Autodesk Inventor part; units mm, degrees
ref_plane "YZ Plane" through (0, 0, 0) normal (1, 0, 0) x (0, 1, 0)
ref_plane "XZ Plane" through (0, 0, 0) normal (0, 1, 0) x (-1, 0, 0)
ref_plane "XY Plane" through (0, 0, 0) normal (0, 0, 1) x (1, 0, 0)
sketch "Эскиз1" plane through (0, 0, 0) normal (0, 1, 0) x (-1, 0, 0)
  line L0 (7, 44) -> (0, 44)
  line L1 (0, 44) -> (0, 0)
  line L2 (0, 0) -> (7, 0)
  line L3 (7, 0) -> (7, 44)
  line L4 (-16.3445, 0) -> (14.925, 0) construction
  line L5 (0, 24.3748) -> (0, -24.0504) construction
  circle A0 centre (3.5, 39) radius 1.75
  line L6 (3.5, 44) -> (3.5, 0) construction
  line L7 (7, 22) -> (0, 22) construction
  circle A1 centre (3.5, 5) radius 1.75
  point P0 (0, 0)
  dimension "d0" = 44
  dimension "d1" = 7
  dimension "d2" = 3.5
  dimension "d5" = 34
extrude "Выдавливание1" add sketch "Эскиз1" along normal blind 30
sketch "Эскиз2" plane through (0, 0, 44) normal (1, 0, 0) x (0, 0, -1)
  line L0 (0, 0) -> (44, 0) construction
  line L1 (44, 0) -> (44, 30) construction
  line L2 (0, 30) -> (44, 30) construction
  line L3 (0, 0) -> (0, 30) construction
  line L4 (44, 30) -> (0, 30) construction
  line L5 (22, 30) -> (22, 0) construction
  line L6 (44, 0) -> (0, 0) construction
  line L7 (0, 0) -> (0, 30) construction
  line L8 (0, 15) -> (44, 15) construction
  line L9 (44, 0) -> (44, 30) construction
  circle A0 centre (22, 11.2) radius 10.25
  circle A1 centre (22, 11.2) radius 3.75
  circle A2 centre (22, 18.7) radius 1.5
  line L10 (18.25, 11.2) -> (25.75, 11.2) construction
  circle A3 centre (22, 3.7) radius 1.5
  dimension "d8" = 20.5
  dimension "d9" = 11.2
  dimension "d10" = 7.5
  dimension "d11" = 3
  dimension "d12" = 15
extrude "Выдавливание2" cut sketch "Эскиз2" against normal blind 30 contours A1 | A2 | A3
extrude "Выдавливание3" cut sketch "Эскиз2" against normal blind 4
properties part number "motor_front"
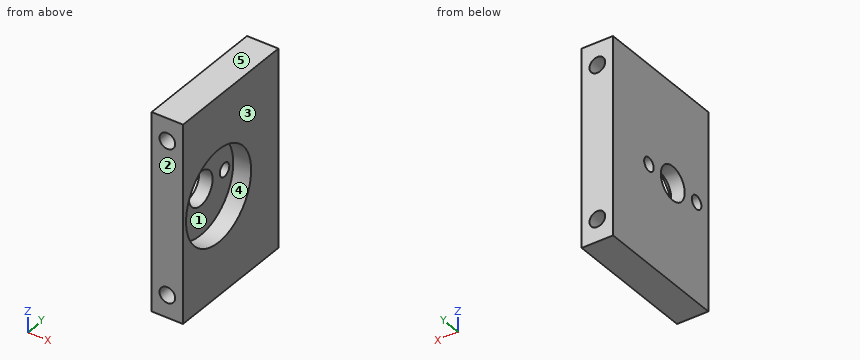
Geometry: final body of the model. Coordinates: model frame, mm. Face numbers are marked on the shaded views. A direction names the side the tool comes from. Give positions to 0.01 mm unless a question says otherwise; leave off trailing zeros. Order: outer loops, then holes, each group sorted by start corner. A loop starts at its lowest first (then second) coordinate and runs counter-clockwise, first axis right, second up. Notation, with made-up numbers: (27.5, 30.5) -> (64.5, 30.5) arc R25 ccw to (64.5, 49.5) -> close; hole circle Ø11 at (0.25, 83.25). An arc over 180 degrees is marked (long way). Write each question's results on one line, items separated by ' | '. Start each with the question number.
1) Section D-D (z = 5). Return loops of the section in (x, y), then the cut area to 3 significant figures.
2) Section C-C (y = 11.2). Return loops of the section in (x, z).
3) Section A-A (x = -3.5). Return loops of the section in (y, z), then the cut area to 3 significant figures.
4) Line query: line 1 (Y direction, x = -4.65, z = 22); line 2 (Z direction, x = -4.5, y = 26.5); line 3 (Y direction, x = -6.25, z = 21). Output: solid intervals per line, ascending. Write a range as from..to.
5) Section B-B (z = 22). Return loops of the section in (x, y), then the cut area to 3 significant figures.
6) Set-up query: the marked faces 4 and 5. Return all of +Z, -Z, +X, -X, +Y, -Y with unobstructed straight access to the full face (end or side cutting, diameter ignored); none if empty.
7) Draft query along Y for the marked faces 1, 2 and 3. Return one class per face: pulls with the +Y half, pulls with the -Y half, needs draft (parallel to the pull), parting line crosses it, or undercut.
8) First-contact query: pin 1 (2 mm diameter, centred on x = -3.5, z = 5, fed in from -Y); pin 2 (4 mm diameter, centred on y = 18.7, z = 22, fed in from +X). Flat tips, straight axial feed; report the tip coordinate or a pass-through.
Calculated:
1) outline: (-7, 0) -> (-5.25, 0) -> (-5.25, 30) -> (-7, 30) -> close; (-1.75, 0) -> (0, 0) -> (0, 30) -> (-1.75, 30) -> close | area: 105 mm2
2) outline: (-7, 0) -> (0, 0) -> (0, 11.75) -> (-4, 11.75) -> (-4, 18.25) -> (-7, 18.25) -> close; (-7, 25.75) -> (-4, 25.75) -> (-4, 32.25) -> (0, 32.25) -> (0, 44) -> (-7, 44) -> close; hole circle Ø3.5 at (-3.5, 5); hole circle Ø3.5 at (-3.5, 39)
3) outline: (0, 0) -> (30, 0) -> (30, 3.25) -> (0, 3.25) -> close; (0, 6.75) -> (30, 6.75) -> (30, 37.25) -> (0, 37.25) -> close; (0, 40.75) -> (30, 40.75) -> (30, 44) -> (0, 44) -> close; hole circle Ø20.5 at (11.2, 22) | area: 780 mm2
4) line 1: 0..2.2, 5.2..7.45, 14.95..17.2, 20.2..30 | line 2: 0..3.56, 6.44..37.56, 40.44..44 | line 3: 0..2.58, 4.82..7.59, 14.81..17.58, 19.82..30
5) outline: (-7, 0) -> (0, 0) -> (0, 0.95) -> (-4, 0.95) -> (-4, 2.2) -> (-7, 2.2) -> close; (-7, 5.2) -> (-4, 5.2) -> (-4, 7.45) -> (-7, 7.45) -> close; (-7, 14.95) -> (-4, 14.95) -> (-4, 17.2) -> (-7, 17.2) -> close; (-7, 20.2) -> (-4, 20.2) -> (-4, 21.45) -> (0, 21.45) -> (0, 30) -> (-7, 30) -> close | area: 87.5 mm2
6) face 4: +X | face 5: +Z, +X, -X, +Y, -Y
7) face 1: undercut | face 2: pulls with the -Y half | face 3: needs draft
8) pin 1: through | pin 2: x = -4
